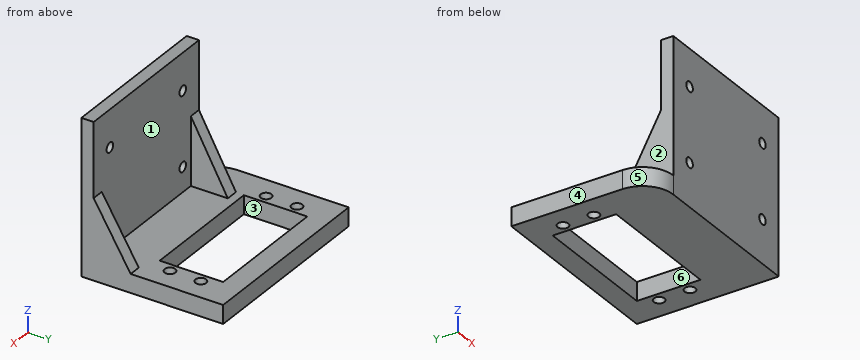
```python
from build123d import *

# Parameters (mm, degrees)
SCHIZZO1_W                    = 62
SCHIZZO1_H                    = 6
ESTRUSIONE_ESTRUSIONE1_DEPTH  = 46
TAGLIO_ESTRUSIONE1_DEPTH      = 56.555261254
TAGLIO_ESTRUSIONE1_DEPTH_BACK = 56.555261254
SCHIZZO3_W                    = 41.6
SCHIZZO3_H                    = 20.6
SCHIZZO6_R                    = 1.75
TAGLIO_ESTRUSIONE2_DEPTH      = 56.794264938
SCHIZZO7_W                    = 52
SCHIZZO7_H                    = 4
ESTRUSIONE_ESTRUSIONE3_DEPTH  = 44
SCHIZZO10_R                   = 1.6
TAGLIO_ESTRUSIONE4_DEPTH      = 71.285162547
ESTRUSIONE_ESTRUSIONE4_DEPTH  = 4
ESTRUSIONE_ESTRUSIONE5_DEPTH  = 4
RACCORDO3_R                   = 10


with BuildPart() as part:
    # Schizzo1 → Estrusione-Estrusione1 (new body)
    with BuildSketch(Plane(origin=(0, 0, 0), x_dir=(1, 0, 0), z_dir=(0, 1, 0))):
        with Locations((0, -0.063829787)):
            Rectangle(SCHIZZO1_W, SCHIZZO1_H)
    extrude(amount=ESTRUSIONE_ESTRUSIONE1_DEPTH)

    # Schizzo3 → Taglio-Estrusione1 (cut, two sides: drawn at the far end of the back side and taken through both)
    with BuildSketch(Plane.XY.offset(-TAGLIO_ESTRUSIONE1_DEPTH_BACK)):
        with Locations((0, 29)):
            Rectangle(SCHIZZO3_W, SCHIZZO3_H)
    extrude(amount=TAGLIO_ESTRUSIONE1_DEPTH + TAGLIO_ESTRUSIONE1_DEPTH_BACK, mode=Mode.SUBTRACT)

    # Schizzo6 → Taglio-Estrusione2 (cut, through all)
    with BuildSketch(Plane.XY.offset(3.063829787)):
        with Locations((-23.75, 34)):
            Circle(SCHIZZO6_R)
        with Locations(Location((-23.75, 24, 0), (0, 0, 180))):
            Circle(SCHIZZO6_R)
        with Locations((23.75, 24)):
            Circle(SCHIZZO6_R)
        with Locations(Location((23.75, 34, 0), (0, 0, 180))):
            Circle(SCHIZZO6_R)
    extrude(amount=-TAGLIO_ESTRUSIONE2_DEPTH, mode=Mode.SUBTRACT)

    # Schizzo7 → Estrusione-Estrusione3 (add)
    with BuildSketch(Plane.XY.offset(3.063829787)):
        with Locations((5, 2)):
            Rectangle(SCHIZZO7_W, SCHIZZO7_H)
    extrude(amount=ESTRUSIONE_ESTRUSIONE3_DEPTH)

    # Schizzo10 → Taglio-Estrusione4 (cut, through all)
    with BuildSketch(Plane(origin=(0, 4, 0), x_dir=(1, 0, 0), z_dir=(0, 1, 0))):
        with Locations(Location((-13, -11.063829787, 0), (0, 0, 180))):
            Circle(SCHIZZO10_R)
        with Locations((-13, -35.063829787)):
            Circle(SCHIZZO10_R)
        with Locations(Location((23, -35.063829787, 0), (0, 0, 180))):
            Circle(SCHIZZO10_R)
        with Locations((23, -11.063829787)):
            Circle(SCHIZZO10_R)
    extrude(amount=-TAGLIO_ESTRUSIONE4_DEPTH, mode=Mode.SUBTRACT)

    # Schizzo13 → Estrusione-Estrusione4 (add)
    with BuildSketch(Plane(origin=(31, 0, 0), x_dir=(0, 0, -1), z_dir=(1, 0, 0))):
        Polygon((-23.063829787, 4), (-3.063829787, 16), (-3.063829787, 4), align=None)
    extrude(amount=-ESTRUSIONE_ESTRUSIONE4_DEPTH)

    # Schizzo15 → Estrusione-Estrusione5 (add)
    with BuildSketch(Plane.ZY.offset(21)):
        Polygon((25.063829787, 4), (3.063829787, 4), (3.063829787, 16), align=None)
    extrude(amount=-ESTRUSIONE_ESTRUSIONE5_DEPTH)

    # Raccordo3
    raccordo3_edges = [part.edges().sort_by_distance(p)[0] for p in [
        (-31, 0, 0.063829787),
    ]]
    fillet(raccordo3_edges, radius=RACCORDO3_R)


solid = part.part
```
Input: part model. Units: mm. Frame: model coordinates. Face numbers are marked on the shaded views. A direction names the side the tool comes from. Coordinates: 2 decimals unless noted, no trailing zeros. Loops run counter-clockwise (first coordinate to the right, second up) from the corner with the lowest first, then second, coordinate; pieces in that order, holes last. Notation, with made-up numbers: (52.25, 72) -> (57.25, 72) arc R29 cw to (57.25, 108) -> close; hole circle Ø4 at (-30, 84). An arc over 180 degrees is marked (long way). Use a Markdown table: item, result.
1) Cut plane A-A (x = 15.5). Return the cut outline in (y, z), then the cut area to 3 significant figures.
Results found:
| item | result |
|---|---|
| outline | (0, -2.94) -> (18.7, -2.94) -> (18.7, 3.06) -> (4, 3.06) -> (4, 47.06) -> (0, 47.06) -> close; (39.3, -2.94) -> (46, -2.94) -> (46, 3.06) -> (39.3, 3.06) -> close |
| area | 328 mm2 |
2) Access query for the marked faces 1, 2 and 3. Directions: +Z, -Z, +X, -X, +Y, -Y. A direction counts if a zero-diameter tool reaches every point of the face in a straight line with its end or side. Return the directions, or none.
Results found:
| item | result |
|---|---|
| face 1 | +Z, +Y |
| face 2 | +Z, -X, +Y, -Y |
| face 3 | +Z, -Z |
3) Cut plane B-B (y = 21). Return the cut outline in (x, z), then the cut area to 3 significant figures.
Results found:
| item | result |
|---|---|
| outline | (-31, -2.94) -> (-20.8, -2.94) -> (-20.8, 3.06) -> (-31, 3.06) -> close; (20.8, -2.94) -> (31, -2.94) -> (31, 3.06) -> (20.8, 3.06) -> close |
| area | 122 mm2 |
4) Cut plane D-D (x = 23.75). Return the cut outline in (y, z), then the cut area to 3 significant figures.
Results found:
| item | result |
|---|---|
| outline | (0, -2.94) -> (22.25, -2.94) -> (22.25, 3.06) -> (4, 3.06) -> (4, 9.65) -> (0, 9.65) -> close; (0, 12.48) -> (4, 12.48) -> (4, 33.65) -> (0, 33.65) -> close; (0, 36.48) -> (4, 36.48) -> (4, 47.06) -> (0, 47.06) -> close; (25.75, -2.94) -> (32.25, -2.94) -> (32.25, 3.06) -> (25.75, 3.06) -> close; (35.75, -2.94) -> (46, -2.94) -> (46, 3.06) -> (35.75, 3.06) -> close |
| area | 387 mm2 |
5) Pull-direction query (Y, two-part tool) for the marked faces 4, 5 and 6; classes: released by +Y, released by -Y, zero draft, split by the parting line, or undercut.
Results found:
| item | result |
|---|---|
| face 4 | zero draft |
| face 5 | released by -Y |
| face 6 | undercut |
6) Cut plane C-C (y = 34). Return the cut outline in (x, z).
Results found:
| item | result |
|---|---|
| outline | (-31, -2.94) -> (-25.5, -2.94) -> (-25.5, 3.06) -> (-31, 3.06) -> close; (-22, -2.94) -> (-20.8, -2.94) -> (-20.8, 3.06) -> (-22, 3.06) -> close; (20.8, -2.94) -> (22, -2.94) -> (22, 3.06) -> (20.8, 3.06) -> close; (25.5, -2.94) -> (31, -2.94) -> (31, 3.06) -> (25.5, 3.06) -> close |
7) Contact query for flat-ended pins moving along their axis: pin 1 (22 mm diameter, centred on x = 15, z = 19.5, fed in from +Y); pin 2 (1 mm diameter, centred on x = -13.5, y = 9, fed in from +Z); pin 3 (17.5 mm diameter, centred on y = 4.5, z = 16.5, fed in from -X). Output: stop coordinate, or through.
Results found:
| item | result |
|---|---|
| pin 1 | stops at y = 4 |
| pin 2 | stops at z = 3.06 |
| pin 3 | stops at x = -21 |
8) Material intervals for line 1 along Y through (x, z) = (23.75, -0.2); line 2 along Z through (x, y) = (23, 3); line 3 along Y through (x, z) = (-19.5, 32), sorted ascending. Write a range as from..to.
Results found:
| item | result |
|---|---|
| line 1 | y = 0..22.25, 25.75..32.25, 35.75..46 |
| line 2 | z = -2.94..9.46, 12.66..33.46, 36.66..47.06 |
| line 3 | y = 0..4 |
